Here's how the part is built. I have some questions about the finished solid (model axes, mm). A direction names the side the tool comes from. Give positions to 0.01 mm unless a question says otherwise; leave off trailing zeros. Order: outer loops, then holes, each group sorted by start corner. A loop starts at its lowest first (then second) coordinate and runs counter-clockwise, first axis right, second up.
from build123d import *

# Parameters (mm, degrees)
F1_DEPTH  = 6.1214
F2_W      = 126.3396
F2_H      = 43.2846567154
F3_DEPTH  = 1.2446
F4_W      = 85.1099437237
F4_H      = 19.05
F5_DEPTH  = 0.5842
F7_DEPTH  = 5.5372
F8_R      = 1.8923
F9_DEPTH  = 4.8768
F10_R     = 1.8923
F11_DEPTH = 5.5372
F12_R     = 3.2639
F13_DEPTH = 6.1214
F14_R     = 1.8923
F15_DEPTH = 5.5372
F16_R     = 3.2639
F17_DEPTH = 5.5372


with BuildPart() as f1:
    # F0 (on Top) → F1 (new body)
    with BuildSketch(Plane.XY):
        Polygon((0, 51.1556), (0, 0), (126.3396, 0), (126.3396, 51.1556), (117.2718, 51.1556), (117.2718, 60.6806), (107.7468, 60.6806), (107.7468, 51.1556), (73.787, 51.1556), (73.787, 60.6806), (64.262, 60.6806), (64.262, 51.1556), align=None)
    extrude(amount=F1_DEPTH)

    # F2 (on face) → F3 (cut)
    with BuildSketch(Plane.XY.offset(6.1214)):
        with Locations((63.1698, 40.6923283577)):
            Rectangle(F2_W, F2_H)
    extrude(amount=-F3_DEPTH, mode=Mode.SUBTRACT)

    # F4 (on face) → F5 (cut)
    with BuildSketch(Plane.XY.offset(6.1214)):
        with Locations((83.8299718618, 9.525)):
            Rectangle(F4_W, F4_H)
    extrude(amount=-F5_DEPTH, mode=Mode.SUBTRACT)

    # F6 (on face) → F7 (cut, through all)
    with BuildSketch(Plane.XY.offset(5.5372)):
        with BuildLine():
            Line((74.6125, 19.05), (44.45, 19.05))
            ThreePointArc((44.45, 19.05), (41.275, 15.875), (44.45, 12.7))
            Line((44.45, 12.7), (74.6125, 12.7))
            ThreePointArc((74.6125, 12.7), (77.7875, 15.875), (74.6125, 19.05))
        make_face()
    extrude(amount=-F7_DEPTH, mode=Mode.SUBTRACT)

    # F8 (on face) → F9 (cut, through all)
    with BuildSketch(Plane.XY.offset(4.8768)):
        with Locations((69.0245, 55.9181)):
            Circle(F8_R)
        with Locations((112.5855, 55.9181)):
            Circle(F8_R)
    extrude(amount=-F9_DEPTH, mode=Mode.SUBTRACT)

    # F10 (on face) → F11 (cut, through all)
    with BuildSketch(Plane.XY.offset(5.5372)):
        with Locations((59.53125, 6.35)):
            Circle(F10_R)
    extrude(amount=-F11_DEPTH, mode=Mode.SUBTRACT)

    # F12 (on face) → F13 (cut, through all)
    with BuildSketch(Plane.XY.offset(6.1214)):
        with Locations((9.525, 6.731)):
            Circle(F12_R)
    extrude(amount=-F13_DEPTH, mode=Mode.SUBTRACT)

    # F14 (on face) → F15 (cut, through all)
    with BuildSketch(Plane.XY.offset(5.5372)):
        with Locations((85.725, 6.731)):
            Circle(F14_R)
        with Locations((101.6, 6.731)):
            Circle(F14_R)
    extrude(amount=-F15_DEPTH, mode=Mode.SUBTRACT)

    # F16 (on face) → F17 (cut, through all)
    with BuildSketch(Plane.XY.offset(5.5372)):
        with Locations((117.475, 6.731)):
            Circle(F16_R)
    extrude(amount=-F17_DEPTH, mode=Mode.SUBTRACT)


solid = f1.part
Q1. I'm going to push flat-ended pins straight in: P1, Ø1.5, axis at x = 97, z = 1.5, coming from the +Y side; P2, Ø10, axis at x = 61, y = 24, coming from the +Z side; P3, Ø1.5, axis at y = 56, z = 2, coming from the +X side. Where does each tip first touch, or does it pass through?
Filled sheet:
P1: stops at y = 51.16
P2: stops at z = 4.88
P3: stops at x = 117.27
Q2. Thinking about a two-plate mould opening in Y: for faces 4 (the face through (91, 51.156, 2)), 5 (the face through (117.272, 56, 2)), 6 (the face through (59.285, 8.226, 2.807)), which applies, released by +Y, released by -Y, zero draft, split by the parting line, or undercut?
Filled sheet:
face 4: released by +Y
face 5: zero draft
face 6: undercut
Q3. I need wall thicknesses on L1, parallel to Y at x = 101.6, z = 4.4; L2, parallel to Y at x = 48.5, z = 3.25; L3, parallel to Z at x = 59, y = 23.5. Which ranges of each line are inside material? Lowest first, please.
Filled sheet:
L1: y = 0 to 4.84, 8.62 to 51.16
L2: y = 0 to 12.7, 19.05 to 51.16
L3: z = 0 to 4.88
Q4. For faces 1 (the face through (33, 51.156, 2)), 2 (the face through (41.276, 15.945, 2.807)), 3 (the face through (73.787, 56, 2)), which set-ups out of +Z, -Z, +X, -X, +Y, -Y let a thin tool reach every point of the face, with its end or its side?
Filled sheet:
face 1: +Z, -Z, -X, +Y
face 2: +Z, -Z
face 3: +Z, -Z, +Y
Q5. If we section it at C-C on z = 1: Give the number of separate pieces and of enclosed holes in the cut face, plus the area to 3 significant figures.
Filled sheet:
separate pieces: 1
enclosed holes: 8
area: 6,300 mm2
Q6. If we section it at B-B on x = 23: List the corners of the cut face in (y, z) for me.
Filled sheet:
outline: (0, 0) - (51.16, 0) - (51.16, 4.88) - (19.05, 4.88) - (19.05, 6.12) - (0, 6.12) - close
Q7. If we section it at D-D on x = 101.6: List the corners of the cut face in (y, z) for me, plus the area to 3 significant figures.
Filled sheet:
outline: (0, 0) - (4.84, 0) - (4.84, 5.54) - (0, 5.54) - close; (8.62, 0) - (51.16, 0) - (51.16, 4.88) - (19.05, 4.88) - (19.05, 5.54) - (8.62, 5.54) - close
area: 241 mm2
Q8. If we section it at A-A on x = 54: List the corners of the cut face in (y, z) for me, plus the area to 3 significant figures.
Filled sheet:
outline: (0, 0) - (12.7, 0) - (12.7, 5.54) - (0, 5.54) - close; (19.05, 0) - (51.16, 0) - (51.16, 4.88) - (19.05, 4.88) - close
area: 227 mm2
